Part model, mm, in its own coordinate system. Face numbers are marked on the shaded views. A direction names the side the tool comes from. Round coordinates to 2 decimals unless told otherwise and drop trailing zeros. Loops run counter-clockwise (first coordinate to the right, second up) from the corner with the lowest first, then second, coordinate; pieces in that order, holes last.
from build123d import *

# Parameters (mm, degrees)
NUT_HEX_EXTRUDE_DEPTH  = 3
HEX_EDGE_CHAMFERS_SIZE = 0.2
NYLON_COLLAR_SKETCH_R  = 2.475
NYLON_COLLAR_DEPTH     = 1
THREAD_BORE_SKETCH_R   = 1.4
THREAD_BORE_CUT_DEPTH  = 6.800502852


with BuildPart() as part:
    # Nut Hex Sketch → Nut Hex Extrude (new body)
    with BuildSketch(Plane.XY):
        Polygon((3.175426481, 0), (1.58771324, 2.75), (-1.58771324, 2.75), (-3.175426481, 0), (-1.58771324, -2.75), (1.58771324, -2.75), align=None)
    extrude(amount=NUT_HEX_EXTRUDE_DEPTH)

    # Hex Edge Chamfers
    hex_edge_chamfers_edges = [part.edges().sort_by_distance(p)[0] for p in [
        (0, 2.75, 3),
        (-2.38156986, 1.375, 3),
        (-2.38156986, -1.375, 3),
        (0, -2.75, 3),
        (2.38156986, -1.375, 3),
        (0, -2.75, 0),
        (-2.38156986, -1.375, 0),
        (-2.38156986, 1.375, 0),
        (0, 2.75, 0),
        (2.38156986, 1.375, 0),
        (2.38156986, -1.375, 0),
        (2.38156986, 1.375, 3),
    ]]
    chamfer(hex_edge_chamfers_edges, length=HEX_EDGE_CHAMFERS_SIZE)

    # Nylon Collar Sketch → Nylon Collar (add)
    with BuildSketch(Plane.XY.offset(3)):
        Circle(NYLON_COLLAR_SKETCH_R)
    extrude(amount=NYLON_COLLAR_DEPTH)

    # Thread Bore Sketch → Thread Bore Cut (cut, through all)
    with BuildSketch(Plane.XY):
        Circle(THREAD_BORE_SKETCH_R)
    extrude(amount=THREAD_BORE_CUT_DEPTH, mode=Mode.SUBTRACT)


solid = part.part
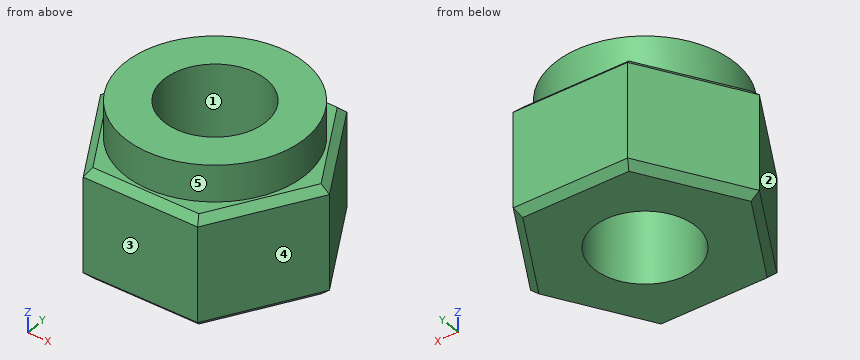
1) Slice it at B-B, the plane z = 2.7. Give the cut face in (x, y), then the cut area to 3 significant figures.
Values:
outline: (-3.18, 0) - (-1.59, -2.75) - (1.59, -2.75) - (3.18, 0) - (1.59, 2.75) - (-1.59, 2.75) - close; hole circle Ø2.8 at (0, 0)
area: 20.0 mm2
2) Mould opens along X. For the marked faces 1, 2 and 3 say: released by +X, released by -X, zero draft, split by the parting line, or undercut.
Values:
face 1: undercut
face 2: released by -X
face 3: zero draft
3) Slice it at D-D, the plane y = 2. Give the cut face in (x, z), then the cut area to 3 significant figures.
Values:
outline: (-2.02, 0.2) - (-1.79, 0) - (1.79, 0) - (2.02, 0.2) - (2.02, 2.8) - (1.79, 3) - (1.46, 3) - (1.46, 4) - (-1.46, 4) - (-1.46, 3) - (-1.79, 3) - (-2.02, 2.8) - close
area: 14.9 mm2
4) Tool access for the marked faces 4 and 5: list every direction of +Z, -Z, +X, -X, +Y, -Y with a clear straight run to the whole face (end or side of a thin tool).
Values:
face 4: +Z, -Z, +X, -Y
face 5: +Z
5) Slice it at A-A, the plane x = 0. Give the cut face in (y, z) (3 decimals).
Values:
outline: (-2.75, 0.2) - (-2.55, 0) - (-1.4, 0) - (-1.4, 4) - (-2.475, 4) - (-2.475, 3) - (-2.55, 3) - (-2.75, 2.8) - close; (1.4, 0) - (2.55, 0) - (2.75, 0.2) - (2.75, 2.8) - (2.55, 3) - (2.475, 3) - (2.475, 4) - (1.4, 4) - close
6) Wall check: line 1 along Y through (x, z) = (0, 0.4); line 2 along Y through (x, z) = (0, 3.2) (3 decimals); line 3 along X through (y, z) = (1, 2.95). Give the ranges that are in metal, low to high.
Values:
line 1: y = -2.75 to -1.4, 1.4 to 2.75
line 2: y = -2.475 to -1.4, 1.4 to 2.475
line 3: x = -2.42 to -0.98, 0.98 to 2.42
7) Drop flat-ended pins along their axis: pin 1 Ø1 at (y, z) = (-1.5, 1.5) entering from +X; pin 2 Ø1.5 at (y, z) = (1, 1) entering from -X; pin 3 Ø1 at (x, z) = (-2, 3.5) entering from -Y. Give the stop position or say it passes through.
Values:
pin 1: stops at x = 2.6
pin 2: stops at x = -3.03
pin 3: stops at y = -1.97
8) Slice it at C-C, the plane y = 0.9. Give the cut face in (x, z), then the cut area to 3 significant figures.
Values:
outline: (-2.66, 0.2) - (-2.42, 0) - (-1.07, 0) - (-1.07, 4) - (-2.31, 4) - (-2.31, 3) - (-2.42, 3) - (-2.66, 2.8) - close; (1.07, 0) - (2.42, 0) - (2.66, 0.2) - (2.66, 2.8) - (2.42, 3) - (2.31, 3) - (2.31, 4) - (1.07, 4) - close
area: 11.9 mm2
